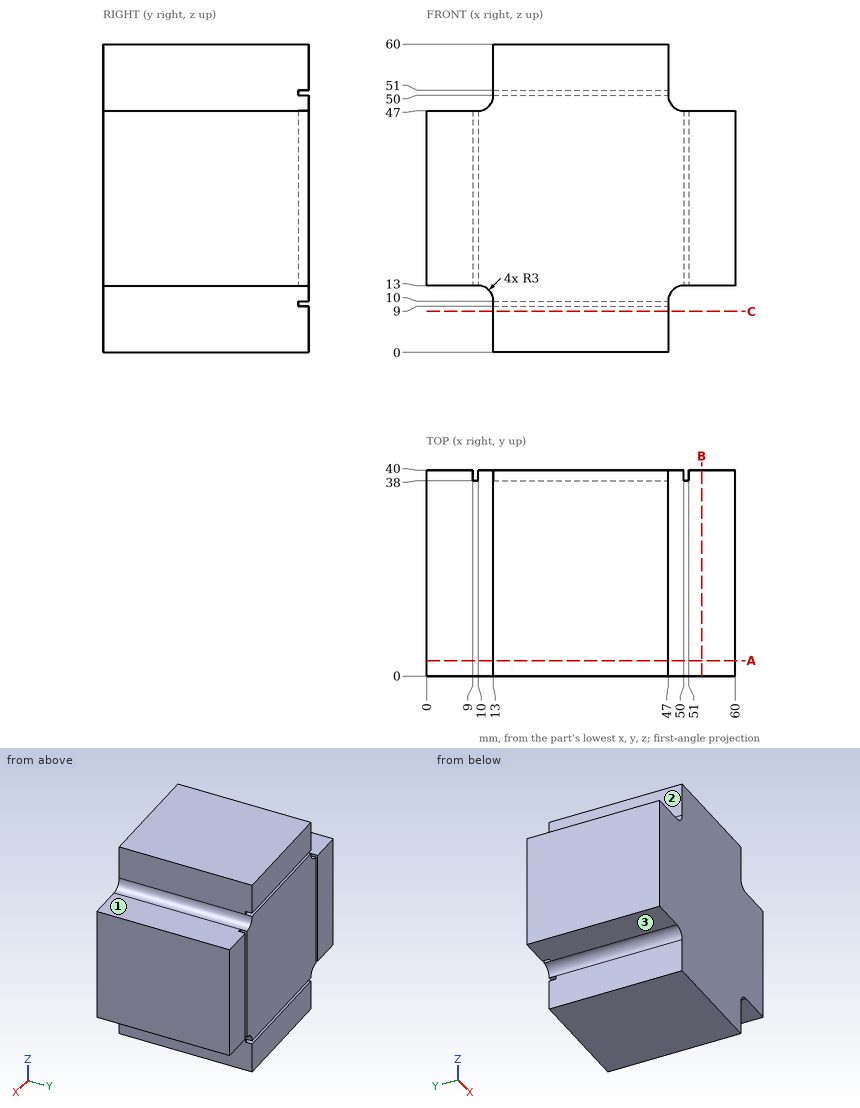
Geometry: see drawing. Coordinates: mm, zero at the bounding-box minimum. A direction names the side the tool comes from. Give positions to 0.01 mm unless a question says otherwise; leave off trailing zeros. Loops run counter-clockwise (first coordinate to the right, second up) from the corner with the lowest first, then second, coordinate; pieces in that order, holes last. Notation, with made-up numbers: (-14, -33) - (-8, -33) arc R7 cw to (-8, -26) - close; hole circle Ø7 at (19.5, 16.25). An arc over 180 degrees is marked (long way). One line per question, with ' | ' between items. Start each with the question number.
(1) Contact query for flat-ended pins moving along their axis: pin 1 (11 mm diameter, centred on x = 56, y = 13.5, fed in from +Z); pin 2 (5 mm diameter, centred on x = 4.5, y = 24.5, fed in from -Z); pin 3 (11 mm diameter, centred on y = 20.5, z = 57, fed in from -X). Output: stop coordinate, or through.
(2) Section query B-B on x = 53.5. Return loops of the section in (y, z), then the cut area to 3 significant figures.
(3) Section query C-C on z = 8. Return loops of the section in (x, y).
(4) Ray query, line 1 (Z direction, x = 2, y = 22.5). Return the intervals inside material, ascending. Write a range as from..to.
(5) Reachability of the marked faces 1, 2 and 3 from +Z, -Z, +X, -X, +Y, -Y: full face, straight path, thin tool, end or side. Return the list, or none.
(6) Section query A-A on y = 3. Return loops of the section in (x, z).
The answers:
1) pin 1: z = 47 | pin 2: z = 13 | pin 3: x = 13
2) outline: (0, 13) - (40, 13) - (40, 47) - (0, 47) - close | area: 1,360 mm2
3) outline: (13, 0) - (47, 0) - (47, 40) - (13, 40) - close
4) line 1: 13..47
5) face 1: +Z, +X, +Y, -Y | face 2: +Z, -X, +Y, -Y | face 3: -Z, -X, +Y, -Y
6) outline: (0, 13) - (10, 13) arc R3 cw to (13, 10) - (13, 0) - (47, 0) - (47, 10) arc R3 cw to (50, 13) - (60, 13) - (60, 47) - (50, 47) arc R3 cw to (47, 50) - (47, 60) - (13, 60) - (13, 50) arc R3 cw to (10, 47) - (0, 47) - close
